Geometry: final body of the model. Coordinates: model frame, mm. A direction names the side the tool comes from. Give positions to 0.01 mm unless a question says otherwise; leave off trailing zeros. Write each loop counter-clockwise with the first axis right and the second up, starting at its lowest first coordinate (ties: lowest second). Pieces come first, ordered by that corner, then holes.
Q1. Line query: line 1 (X direction, y = -3.85, z = 3.5); line 2 (Z direction, x = -15, y = -0.8); line 3 (Y direction, x = -36, z = 1.5). Output: solid intervals per line, ascending.
Q2. Section A-A (x = -5). Return the cut outline in (y, z).
Q3. Reachability of faces 1 (the cylindrical face through (-16.5, -0.99, 6.57)), 2 (the flat face through (-26, -2, 0)), 3 (the flat face through (26, -2, 0)), 4 (the flat face through (0, -3, -0.5)) from +Z, -Z, +X, -X, +Y, -Y: full face, straight path, thin tool, end or side. Return the list, or none.
Q4. Section C-C (x = 15). Return the cut outline in (y, z).
Q5. Mould query, pull axis X, two halves, no side actions, for faces 5 (the cylindrical face through (13.5, -0.99, 6.57)), 6 (the flat face through (-26, -1, -12.5)), 7 (the flat face through (42, -1, 0)), 8 (the flat face through (-10.5, -1, -6)). Classes: +X half, -X half, draft (parallel to the pull), parting line (faces both ways), or undercut.
Q6. Section D-D (x = 29). Return the cut outline in (y, z).
Q7. Pin query (flat end, axial travel): pin 1 Ø3.5 at (x, y) = (-3.5, -2) entering from -Z; pin 2 Ø2.5 at (y, z) = (-4.5, 4.5) entering from +X; pin 3 Ø1 at (x, y) = (-18.5, -3) entering from +Z; pin 4 Ø7.5 at (x, z) = (25.5, 6) entering from -Y. Return the tip coordinate at first contact, or that it passes through.
Q8. Section B-B (y = -3.85). Return the cut outline in (x, z), plus the area to 3 significant figures.
from build123d import *

# Parameters (mm, degrees)
SKETCH_R     = 1.5
PAD_DEPTH    = 2
SKETCH001_W  = 21
SKETCH001_H  = 13
PAD001_DEPTH = 4.85
SKETCH002_R  = 1.5
POCKET_DEPTH = 21


with BuildPart() as part:
    # Sketch → Pad (new body)
    with BuildSketch(Plane.XZ):
        Polygon((-42, 12.5), (42, 12.5), (42, -12.5), (10.5, -12.5), (10.5, -0.5), (-10.5, -0.5), (-10.5, -12.5), (-42, -12.5), align=None)
        with Locations((-15, 6.5)):
            Circle(SKETCH_R, mode=Mode.SUBTRACT)
        with Locations((-15, -6.5)):
            Circle(SKETCH_R, mode=Mode.SUBTRACT)
        with Locations((15, -6.5)):
            Circle(SKETCH_R, mode=Mode.SUBTRACT)
        with Locations((15, 6.5)):
            Circle(SKETCH_R, mode=Mode.SUBTRACT)
    extrude(amount=PAD_DEPTH)

    # Sketch001 (on Face14 of Pad) → Pad001 (join)
    with BuildSketch(Plane.XZ.offset(2)):
        with Locations((0, 6)):
            Rectangle(SKETCH001_W, SKETCH001_H)
    extrude(amount=PAD001_DEPTH)

    # Sketch002 (on Face6 of Pad001) → Pocket (cut)
    with BuildSketch(Plane(origin=(0, 0, 12.5), x_dir=(-1, 0, 0), z_dir=(0, 0, 1))):
        with Locations((-5, 3.85)):
            Circle(SKETCH002_R)
        with Locations((5, 3.85)):
            Circle(SKETCH002_R)
    extrude(amount=-POCKET_DEPTH, mode=Mode.SUBTRACT)


solid = part.part
Computed:
1. line 1: x = -10.5 to -6.5, -3.5 to 3.5, 6.5 to 10.5
1. line 2: z = -12.5 to -8, -5 to 5, 8 to 12.5
1. line 3: y = -2 to 0
2. outline: (-6.85, -0.5) - (-5.35, -0.5) - (-5.35, 12.5) - (-6.85, 12.5) - close; (-2.35, -0.5) - (0, -0.5) - (0, 12.5) - (-2.35, 12.5) - close
3. face 1: +Y, -Y
3. face 2: +Z, -Z, -X, -Y
3. face 3: +Z, -Z, +X, -Y
3. face 4: -Z, +Y, -Y
4. outline: (-2, -12.5) - (0, -12.5) - (0, -8) - (-2, -8) - close; (-2, -5) - (0, -5) - (0, 5) - (-2, 5) - close; (-2, 8) - (0, 8) - (0, 12.5) - (-2, 12.5) - close
5. face 5: undercut
5. face 6: draft
5. face 7: +X half
5. face 8: undercut
6. outline: (-2, -12.5) - (0, -12.5) - (0, 12.5) - (-2, 12.5) - close
7. pin 1: stops at z = -0.5
7. pin 2: stops at x = 10.5
7. pin 3: passes through
7. pin 4: stops at y = -2
8. outline: (-10.5, -0.5) - (-6.5, -0.5) - (-6.5, 12.5) - (-10.5, 12.5) - close; (-3.5, -0.5) - (3.5, -0.5) - (3.5, 12.5) - (-3.5, 12.5) - close; (6.5, -0.5) - (10.5, -0.5) - (10.5, 12.5) - (6.5, 12.5) - close
8. area: 195 mm2
